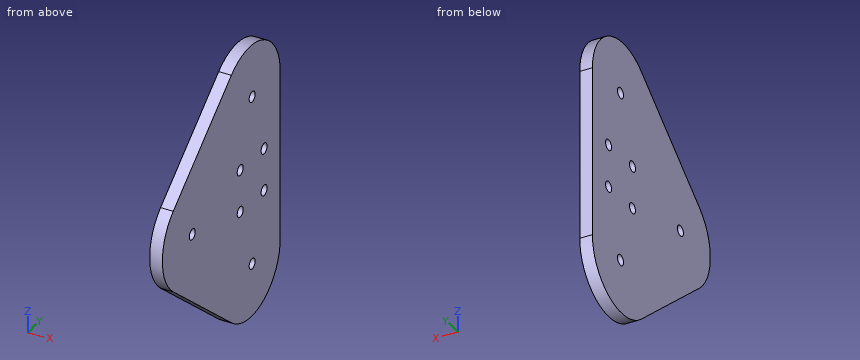
Autodesk Inventor part; units mm, degrees
ref_plane "Work Plane1" through (6, 0, 0) normal (1, 0, 0) x (0, 0, -1)
ref_plane "Work Plane2" through (6, 0, 0) normal (1, 0, 0) x (0, 0, -1)
ref_plane "YZ Plane" through (0, 0, 0) normal (1, 0, 0) x (0, 1, 0)
sketch "Sketch1" plane through (0, 0, 0) normal (1, 0, 0) x (0, 1, 0)
  arc A0 (73.6, 40) -> (32.7129, 59.3028) centre (48.6, 40) ccw
  arc A1 (32.7129, -59.3028) -> (73.6, -40) centre (48.6, -40) ccw
  arc A2 (-15.8871, 19.3028) -> (-15.8871, -19.3028) centre (0, 0) ccw
  line L0 (32.7129, 59.3028) -> (-15.8871, 19.3028)
  line L1 (-15.8871, -19.3028) -> (32.7129, -59.3028)
  line L2 (73.6, -40) -> (73.6, 40)
  dimension "d0" = 80
  dimension "d1" = 48.6
  dimension "d2" = 48.6
  dimension "d3" = 40
  dimension "d4" = 50
  dimension "d5" = 50
  dimension "d6" = 50
ref_plane "Work Plane1" through (6, 0, 0) normal (1, 0, 0) x (0, 0, -1)
sketch "Sketch2" plane through (6, 0, 0) normal (1, 0, 0) x (0, 0, -1)
  circle A0 centre (-40, 50.1) radius 2.5
  circle A1 centre (40, 50.1) radius 2.5
  circle A2 centre (0, 0) radius 2.5
  arc A3 (-19.5369, -15.5983) -> (19.5369, -15.5983) centre (0, 0) ccw
  line L0 (19.5369, -15.5983) -> (59.5369, 34.5017)
  arc A4 (59.5369, 34.5017) -> (40, 75.1) centre (40, 50.1) ccw
  line L1 (40, 75.1) -> (-40, 75.1)
  arc A5 (-40, 75.1) -> (-59.5369, 34.5017) centre (-40, 50.1) ccw
  line L2 (-59.5369, 34.5017) -> (-19.5369, -15.5983)
  dimension "d9" = 5
  dimension "d10" = 5
  dimension "d11" = 5
ref_plane "Work Plane2" through (6, 0, 0) normal (1, 0, 0) x (0, 0, -1)
sketch "Sketch3" plane through (6, 0, 0) normal (1, 0, 0) x (0, 0, -1)
  circle A0 centre (40, 50.1) radius 2.5
  circle A1 centre (-40, 50.1) radius 2.5
  circle A2 centre (0, 0) radius 2.5
  arc A3 (-19.5369, -15.5983) -> (19.5369, -15.5983) centre (0, 0) ccw
  line L0 (19.5369, -15.5983) -> (59.5369, 34.5017)
  arc A4 (59.5369, 34.5017) -> (40, 75.1) centre (40, 50.1) ccw
  line L1 (40, 75.1) -> (-40, 75.1)
  arc A5 (-40, 75.1) -> (-59.5369, 34.5017) centre (-40, 50.1) ccw
  line L2 (-59.5369, 34.5017) -> (-19.5369, -15.5983)
  circle A6 centre (-10, 40.1) radius 2.5
  circle A7 centre (10, 40.1) radius 2.5
  circle A8 centre (10, 60.1) radius 2.5
  circle A9 centre (-10, 60.1) radius 2.5
  dimension "d14" = 5
  dimension "d15" = 5
  dimension "d16" = 5
  dimension "d17" = 5
  dimension "d18" = 20
  dimension "d19" = 20
  dimension "d20" = 20
  dimension "d21" = 20
  dimension "d22" = 15
  dimension "d24" = 10
  dimension "d25" = 15
  dimension "d28" = 10
extrude "Extrusion4" add sketch "Sketch1" along normal blind 6
extrude "Extrusion5" cut sketch "Sketch3" against normal up to next contours A6 | A7 | A8 | A9
extrude "Extrusion6" cut sketch "Sketch2" against normal up to next contours A0 | A1 | A2
properties part number "Arm_Base-SquareBar-Rev3" material "Bronze, Cast"
Source: CAD feature listing. Evaluate the final solid. Frame: model axes, mm. Give positions to 0.01 mm unless a question says otherwise; leave off trailing zeros. Order: outer loops, then holes, each group sorted by start corner. A loop starts at its lowest first (then second) coordinate and runs counter-clockwise, first axis right, second up. Notation, with made-up numbers: (84, 86.5) -> (130, 86.5) arc R13 ccw to (130, 108.5) -> close; hole circle Ø7 at (55, 40). An arc over 180 degrees is marked (long way). Use a Markdown table: item, result.
Q1. Material intervals for line 1 (Y direction, x = 2.4, z = 10); line 2 (Z direction, x = 2.7, y = 39) (3 decimals); line 3 (Y direction, x = 3.4, z = 0), sorted ascending. Write a range as [from, to].
A:
| item | result |
|---|---|
| line 1 | [-22.91, 37.6], [42.6, 57.6], [62.6, 73.6] |
| line 2 | [-63.083, -12.245], [-7.755, 7.755], [12.245, 63.083] |
| line 3 | [-25, -2.5], [2.5, 73.6] |
Q2. Section B-B (x = 2.4). Return the cut outline in (y, z), and give its area (3 significant figures).
A:
| item | result |
|---|---|
| outline | (-15.89, -19.3) -> (32.71, -59.3) arc R25 ccw to (73.6, -40) -> (73.6, 40) arc R25 ccw to (32.71, 59.3) -> (-15.89, 19.3) arc R25 ccw to start; hole circle Ø5 at (0, 0); hole circle Ø5 at (40.1, -10); hole circle Ø5 at (40.1, 10); hole circle Ø5 at (50.1, -40); hole circle Ø5 at (50.1, 40); hole circle Ø5 at (60.1, -10); hole circle Ø5 at (60.1, 10) |
| area | 8,920 mm^2 |
Q3. First-contact query: P1, Ø2, axis at x = 2.5, z = -33, coming from the -Y side; P2, Ø3, axis at x = 4, y = -5.5, coming from the -Z side; P3, Ø2, axis at x = 1.5, z = -19.5, coming from the -Y side. Flat tips, straight axial feed; report the tip coordinate or a pass-through.
A:
| item | result |
|---|---|
| P1 | y = -0.46 |
| P2 | z = -29.09 |
| P3 | y = -16.82 |
Q4. Section D-D (y = 50.1). Return the cut outline in (x, z), and give its area (3 significant figures).
A:
| item | result |
|---|---|
| outline | (0, -64.95) -> (6, -64.95) -> (6, -42.5) -> (0, -42.5) -> close; (0, -37.5) -> (6, -37.5) -> (6, 37.5) -> (0, 37.5) -> close; (0, 42.5) -> (6, 42.5) -> (6, 64.95) -> (0, 64.95) -> close |
| area | 719 mm^2 |
Q5. Section A-A (z = 0). Return the cut outline in (x, y), and give its area (3 significant figures).
A:
| item | result |
|---|---|
| outline | (0, -25) -> (6, -25) -> (6, -2.5) -> (0, -2.5) -> close; (0, 2.5) -> (6, 2.5) -> (6, 73.6) -> (0, 73.6) -> close |
| area | 562 mm^2 |
Q6. Section C-C (y = 40.1). Return the cut outline in (x, z).
A:
| item | result |
|---|---|
| outline | (0, -63.51) -> (6, -63.51) -> (6, -12.5) -> (0, -12.5) -> close; (0, -7.5) -> (6, -7.5) -> (6, 7.5) -> (0, 7.5) -> close; (0, 12.5) -> (6, 12.5) -> (6, 63.51) -> (0, 63.51) -> close |
